Geometry check sheet. Reference: the model listing, model coordinates, mm. A direction names the side the tool comes from. Round coordinates to 2 decimals unless told otherwise and drop trailing zeros. Order: outer loops, then holes, each group sorted by start corner. A loop starts at its lowest first (then second) coordinate and runs counter-clockwise, first axis right, second up. Notation, with made-up numbers: (40.5, -22.5) - (88.5, -22.5) arc R17 cw to (88.5, 8.5) - close; hole circle Ø3 at (33.25, 1). An arc over 180 degrees is marked (long way). One line per question, with ' | ' between items. Start each with the question number.
Q1. Mould release check, pull along Y, two halves, no side actions. Record for faces 1 (the face through (27, 2.5, -15)), 2 (the face through (2, 2.402, -25)), 3 (the face through (40, 5, -15)), 4 (the face through (1.97, 6.32, -2.76)): +Y half, -Y half, draft (parallel to the pull), parting line (faces both ways), or undercut.
Q2. Sectioned sample at C-C, the plane x = 30. Enter the section's corners in (y, z), then the cut area to 3 significant figures.
Q3. Tool access check on faces 5 (the face through (3, 23, -15)), 6 (the face through (1.97, 6.28, -7.26)), 7 (the face through (4.28, 12.32, -40.49)), 8 (the face through (27, 7.5, -15)). Record the directions out of +Z, -Z, +X, -X, +Y, -Y that give a thin tool (end or side, any length) a straight path to the whole face; none if there is none.
Q4. Sectioned sample at D-D, the plane x = 11. Give the number of separate pieces and of enclosed holes in the cut face, then the cut area to 3 significant figures.
Q5. Material ranges on line 1 along Z through (x, y) = (12.25, 5); line 2 along X through (y, z) = (2.5, -39), recorded low to high.
Q6. Gauge pin test, flat ends, axial feed: P1, Ø10, axis at y = 4.5, z = -34.5, coming from the -X side; P2, Ø8, axis at x = 27, z = -16, coming from the -Y side; P3, Ø4, axis at y = 13, z = -40, coming from the -X side; P4, Ø2.5, axis at y = 4, z = -4.5, coming from the -X side. Record the tip position at first contact, or that the pin passes through.
```python
from build123d import *

# Parameters (mm, degrees)
BOSS_EXTRUDE1_DEPTH = 10
BOSS_EXTRUDE2_DEPTH = 15
SKETCH8_R           = 1.6
CUT_EXTRUDE5_DEPTH  = 60.581876439
FILLET1_R           = 12
SKETCH4_W           = 15
SKETCH4_H           = 45
CUT_EXTRUDE2_DEPTH  = 60.581876439
SKETCH6_W           = 10
SKETCH6_H           = 5
BOSS_EXTRUDE3_DEPTH = 25
CUT_EXTRUDE6_DEPTH  = 4


with BuildPart() as part:
    # Sketch1 → Boss-Extrude1 (new body)
    with BuildSketch(Plane(origin=(0, 0, 0), x_dir=(1, 0, 0), z_dir=(0, 1, 0))):
        with BuildLine():
            Line((0, 0), (30, 0))
            Line((30, 0), (30, 30))
            ThreePointArc((30, 30), (15, 45), (0, 30))
            Line((0, 30), (0, 0))
        make_face()
    extrude(amount=BOSS_EXTRUDE1_DEPTH)

    # Sketch2 → Boss-Extrude2 (add)
    with BuildSketch(Plane(origin=(0, 10, 0), x_dir=(1, 0, 0), z_dir=(0, 1, 0))):
        with BuildLine():
            Line((3, 30), (3, 3))
            Line((3, 3), (3, 0))
            Line((3, 0), (0, 0))
            Line((0, 0), (0, 30))
            ThreePointArc((0, 30), (15, 45), (30, 30))
            Line((30, 30), (30, 0))
            Line((30, 0), (27, 0))
            Line((27, 0), (27, 3))
            Line((27, 3), (27, 30))
            ThreePointArc((27, 30), (15, 42), (3, 30))
        make_face()
    extrude(amount=BOSS_EXTRUDE2_DEPTH)

    # Sketch8 → Cut-Extrude5 (cut, through all)
    with BuildSketch(Plane(origin=(0, 0, 0), x_dir=(0, 0, -1), z_dir=(1, 0, 0))):
        with Locations((5, 5)):
            Circle(SKETCH8_R)
        with Locations((25, 5)):
            Circle(SKETCH8_R)
    extrude(amount=CUT_EXTRUDE5_DEPTH, mode=Mode.SUBTRACT)

    # Fillet1
    fillet1_edges = [part.edges().sort_by_distance(p)[0] for p in [
        (3, 10, -15),
        (27, 10, -15),
        (15, 10, -42),
    ]]
    fillet(fillet1_edges, radius=FILLET1_R - 0.0001)  # a hair under: the kernel refuses the full size

    # Sketch4 → Cut-Extrude2 (cut, through all)
    with BuildSketch(Plane(origin=(0, 25, 0), x_dir=(1, 0, 0), z_dir=(0, 1, 0))):
        with Locations((22.5, 22.5)):
            Rectangle(SKETCH4_W, SKETCH4_H)
    extrude(amount=-CUT_EXTRUDE2_DEPTH, mode=Mode.SUBTRACT)

    # Sketch6 → Boss-Extrude3 (add)
    with BuildSketch(Plane(origin=(15, 0, 0), x_dir=(0, 0, -1), z_dir=(1, 0, 0))):
        with Locations((15, 5)):
            Rectangle(SKETCH6_W, SKETCH6_H)
    extrude(amount=BOSS_EXTRUDE3_DEPTH)

    # Sketch9 → Cut-Extrude6 (cut)
    with BuildSketch(Plane.ZY):
        Polygon((-8, 5), (-6.5, 7.598076211), (-3.5, 7.598076211), (-2, 5), (-3.5, 2.401923789), (-6.5, 2.401923789), align=None)
    cut_extrude6 = extrude(amount=-CUT_EXTRUDE6_DEPTH, mode=Mode.SUBTRACT)

    # Mirror2: Cut-Extrude6 across plane
    add(cut_extrude6.mirror(Plane.XY.offset(-15)), mode=Mode.SUBTRACT)


solid = part.part
```
Determined:
1) face 1: -Y half | face 2: undercut | face 3: draft | face 4: undercut
2) outline: (2.5, -20) - (7.5, -20) - (7.5, -10) - (2.5, -10) - close | area: 50.0 mm2
3) face 5: +Z, +X, +Y | face 6: -X | face 7: -Z, -X, +Y, -Y | face 8: +Z, -Z, +X, +Y
4) separate pieces: 1 | enclosed holes: 2 | area: 531 mm2
5) line 1: z = -44.75 to -26.6, -23.4 to -6.6, -3.4 to 0 | line 2: x = 3 to 15
6) P1: stops at x = 0 | P2: stops at y = 2.5 | P3: stops at x = 2.31 | P4: stops at x = 4
